Design review of the part built by this model. Coordinates are the model's own, in mm. Face numbers are marked on the shaded views. A direction names the side the tool comes from. Round coordinates to 2 decimals unless told otherwise and drop trailing zeros. Order: outer loops, then holes, each group sorted by start corner. A loop starts at its lowest first (then second) coordinate and runs counter-clockwise, first axis right, second up. Notation, with made-up numbers: (-29, 19.5) - (23, 19.5) arc R11 cw to (23, 35.5) - close; hole circle Ø8 at (49.5, 41). An arc over 180 degrees is marked (long way). Write item = value, one per line.
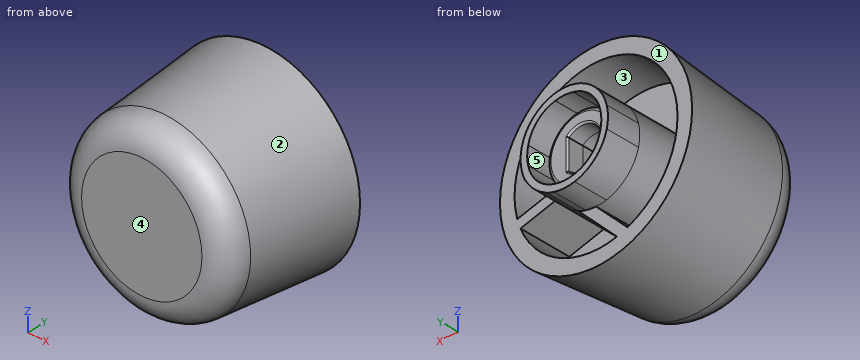
from build123d import *
from build123d.topology import SkipClean

# Parameters (mm, degrees)
SKETCH1_R             = 5
BOSS_EXTRUDE1_DEPTH   = 2.5
BOSS_EXTRUDE2_DEPTH   = 5.2
BOSS_EXTRUDE2_2_DEPTH = 5.2
BOSS_EXTRUDE2_3_DEPTH = 5.2
BOSS_EXTRUDE2_4_DEPTH = 5.2
FILLET1_R             = 0.5
FILLET2_R             = 0.5
FILLET3_R             = 0.5
FILLET4_R             = 0.5
SKETCH3_R             = 14.5
BOSS_EXTRUDE3_DEPTH   = 20
SKETCH4_OUTSIDE_W     = 44.126
SKETCH4_OUTSIDE_H     = 44.126
SKETCH4_OUTSIDE_R     = 14.5
CUT_EXTRUDE2_DEPTH    = 20
CUT_EXTRUDE2_DRAFT    = 5
FILLET5_R             = 4
CUT_EXTRUDE3_START    = -14
CUT_EXTRUDE3_DEPTH    = 14
FILLET6_R             = 0.25
FILLET7_R             = 0.5
CUT_EXTRUDE4_START    = -8
SKETCH6_R             = 12.3
SKETCH6_R_2           = 6.6
CUT_EXTRUDE4_DEPTH    = 8
BOSS_EXTRUDE4_DEPTH   = 8
BOSS_EXTRUDE5_DEPTH   = 5.2


# Read off the part's stored shape, not the designer's step: Boss-Extrude5
with BuildPart() as part:
    # Sketch1 → Boss-Extrude1 (new body)
    with BuildSketch(Plane(origin=(0, 0, 0), x_dir=(1, 0, 0), z_dir=(0, 1, 0))):
        with Locations(Location((0, 0, 0), (0, 0, 270))):
            Circle(SKETCH1_R)
        with BuildLine():
            Line((2, 2.236067977), (2, -2.236067977))
            ThreePointArc((2, -2.236067977), (-3, 0), (2, 2.236067977))
        make_face(mode=Mode.SUBTRACT)
    extrude(amount=BOSS_EXTRUDE1_DEPTH)



with BuildPart() as body_2:
    # Sketch2 → Boss-Extrude2 (new body)
    with BuildSketch(Plane.XZ):
        with BuildLine():
            Line((-6.305354867, 1.95), (-5.249523788, 1.95))
            ThreePointArc((-5.249523788, 1.95), (-5.6, 0), (-5.249523788, -1.95))
            Line((-5.249523788, -1.95), (-6.305354867, -1.95))
            ThreePointArc((-6.305354867, -1.95), (-6.6, 0), (-6.305354867, 1.95))
        make_face()
    extrude(amount=-BOSS_EXTRUDE2_DEPTH)

    # Fillet4
    fillet4_edges = [body_2.edges().sort_by_distance(p)[0] for p in [
        (-6.305354867, 2.6, 1.95),
        (-5.249523788, 2.6, -1.95),
        (-6.305354867, 2.6, -1.95),
        (-5.249523788, 2.6, 1.95),
    ]]
    fillet(fillet4_edges, radius=FILLET4_R - 0.0001)  # a hair under: the kernel refuses the full size


with BuildPart() as body_3:
    # Sketch2 → Boss-Extrude2 2 (new body)
    with BuildSketch(Plane.XZ):
        with BuildLine():
            Line((-1.95, 6.305354867), (-1.95, 5.249523788))
            ThreePointArc((-1.95, 5.249523788), (0, 5.6), (1.95, 5.249523788))
            Line((1.95, 5.249523788), (1.95, 6.305354867))
            ThreePointArc((1.95, 6.305354867), (0, 6.6), (-1.95, 6.305354867))
        make_face()
    extrude(amount=-BOSS_EXTRUDE2_2_DEPTH)

    # Fillet3
    fillet3_edges = [body_3.edges().sort_by_distance(p)[0] for p in [
        (-1.95, 2.6, 6.305354867),
        (-1.95, 2.6, 5.249523788),
        (1.95, 2.6, 6.305354867),
        (1.95, 2.6, 5.249523788),
    ]]
    fillet(fillet3_edges, radius=FILLET3_R - 0.0001)  # a hair under: the kernel refuses the full size


with BuildPart() as body_4:
    # Sketch2 → Boss-Extrude2 3 (new body)
    with BuildSketch(Plane.XZ):
        with BuildLine():
            Line((6.305354867, 1.95), (5.249523788, 1.95))
            ThreePointArc((5.249523788, 1.95), (5.6, 0), (5.249523788, -1.95))
            Line((5.249523788, -1.95), (6.305354867, -1.95))
            ThreePointArc((6.305354867, -1.95), (6.6, 0), (6.305354867, 1.95))
        make_face()
    extrude(amount=-BOSS_EXTRUDE2_3_DEPTH)

    # Fillet2
    fillet2_edges = [body_4.edges().sort_by_distance(p)[0] for p in [
        (6.305354867, 2.6, 1.95),
        (6.305354867, 2.6, -1.95),
        (5.249523788, 2.6, -1.95),
        (5.249523788, 2.6, 1.95),
    ]]
    fillet(fillet2_edges, radius=FILLET2_R - 0.0001)  # a hair under: the kernel refuses the full size


with BuildPart() as body_5:
    # Sketch2 → Boss-Extrude2 4 (new body)
    with BuildSketch(Plane.XZ):
        with BuildLine():
            Line((1.95, -6.305354867), (1.95, -5.249523788))
            ThreePointArc((1.95, -5.249523788), (0, -5.6), (-1.95, -5.249523788))
            Line((-1.95, -5.249523788), (-1.95, -6.305354867))
            ThreePointArc((-1.95, -6.305354867), (0, -6.6), (1.95, -6.305354867))
        make_face()
    extrude(amount=-BOSS_EXTRUDE2_4_DEPTH)

    # Fillet1
    fillet1_edges = [body_5.edges().sort_by_distance(p)[0] for p in [
        (1.95, 2.6, -6.305354867),
        (-1.95, 2.6, -6.305354867),
        (1.95, 2.6, -5.249523788),
        (-1.95, 2.6, -5.249523788),
    ]]
    fillet(fillet1_edges, radius=FILLET1_R - 0.0001)  # a hair under: the kernel refuses the full size


with BuildPart() as part_1:
    add(part.part)

    add(body_2.part)  # Boss-Extrude3 merges body 2

    add(body_3.part)  # Boss-Extrude3 merges body 3

    add(body_4.part)  # Boss-Extrude3 merges body 4

    add(body_5.part)  # Boss-Extrude3 merges body 5
    # Sketch3 → Boss-Extrude3 (add)
    with BuildSketch(Plane(origin=(0, 0, 0), x_dir=(1, 0, 0), z_dir=(0, 1, 0))):
        with Locations(Location((0, 0, 0), (0, 0, 270))):
            Circle(SKETCH3_R)
    extrude(amount=-BOSS_EXTRUDE3_DEPTH)


with BuildPart() as cut_extrude2_tool:
    # Sketch4 outside → Cut-Extrude2 (with draft: the straight prism first)
    with BuildSketch(Plane(origin=(0, 0, 0), x_dir=(1, 0, 0), z_dir=(0, 1, 0))):
        Rectangle(SKETCH4_OUTSIDE_W, SKETCH4_OUTSIDE_H)
        Circle(SKETCH4_OUTSIDE_R, mode=Mode.SUBTRACT)
    extrude(amount=-CUT_EXTRUDE2_DEPTH)
    # Cut-Extrude2: the draft: its side faces are tilted about the plane it starts from
    cut_extrude2_sides = [cut_extrude2_tool.faces().sort_by_distance(p)[0] for p in [
        (0, -10, 22.063),
        (22.063, -10, 0),
        (0, -10, -22.063),
        (-22.063, -10, 0),
        (-14.5, -10, 0),
    ]]
    draft(cut_extrude2_sides, Plane(origin=(0, 0, 0), x_dir=(1, 0, 0), z_dir=(0, 1, 0)), CUT_EXTRUDE2_DRAFT)


with BuildPart() as part_2:
    add(part_1.part)

    # Cut-Extrude2: cut by cut_extrude2_tool
    add(cut_extrude2_tool.part, mode=Mode.SUBTRACT)

    # Fillet5
    fillet5_edges = [part_2.edges().sort_by_distance(p)[0] for p in [
        (-12.750226729, -20, 0),
    ]]
    fillet(fillet5_edges, radius=FILLET5_R)

    # Sketch5 → Cut-Extrude3 (cut)
    with SkipClean():  # the faces are left unmerged after this step: merging them gives an invalid solid
        with BuildSketch(Plane(origin=(0, 0, 0), x_dir=(1, 0, 0), z_dir=(0, 1, 0)).offset(CUT_EXTRUDE3_START)):
            with BuildLine():
                Line((2, -2.236067977), (2, 2.236067977))
                ThreePointArc((2, 2.236067977), (-3, 0), (2, -2.236067977))
            make_face()
        extrude(amount=CUT_EXTRUDE3_DEPTH, mode=Mode.SUBTRACT)

    # Fillet6
    fillet6_edges = [part_2.edges().sort_by_distance(p)[0] for p in [
        (-3, 2.5, 0),
        (2, 2.5, 0),
    ]]
    fillet(fillet6_edges, radius=FILLET6_R)

    # Fillet7
    fillet7_edges = [part_2.edges().sort_by_distance(p)[0] for p in [
        (0, 2.5, -5),
    ]]
    fillet(fillet7_edges, radius=FILLET7_R)

    # Sketch6 → Cut-Extrude4 (cut)
    with SkipClean():  # the faces are left unmerged after this step: merging them gives an invalid solid
        with BuildSketch(Plane(origin=(0, 0, 0), x_dir=(1, 0, 0), z_dir=(0, 1, 0)).offset(CUT_EXTRUDE4_START)):
            with Locations(Location((0, 0, 0), (0, 0, 270))):
                Circle(SKETCH6_R)
            with Locations(Location((0, 0, 0), (0, 0, 76.248877743))):
                Circle(SKETCH6_R_2, mode=Mode.SUBTRACT)
        extrude(amount=CUT_EXTRUDE4_DEPTH, mode=Mode.SUBTRACT)

    # Sketch7 → Boss-Extrude4 (add)
    with SkipClean():  # the faces are left unmerged after this step: merging them gives an invalid solid
        with BuildSketch(Plane(origin=(0, -8, 0), x_dir=(1, 0, 0), z_dir=(0, 1, 0))):
            with BuildLine():
                Line((6.375110454, 1.708205698), (11.880887663, 3.183474255))
                ThreePointArc((11.880887663, 3.183474255), (11.664219973, 3.903328376), (11.40398128, 4.608601845))
                Line((11.40398128, 4.608601845), (5.820052572, 3.112392657))
                ThreePointArc((5.820052572, 3.112392657), (6.137868976, 2.426224317), (6.375110454, 1.708205698))
            make_face()
            with BuildLine():
                Line((2.697938648, 6.023381696), (-3.164606791, 11.885927135))
                ThreePointArc((-3.164606791, 11.885927135), (-3.964993354, 11.643402754), (-4.747049149, 11.347049149))
                Line((-4.747049149, 11.347049149), (0, 6.6))
                ThreePointArc((0, 6.6), (1.379434813, 6.454235787), (2.697938648, 6.023381696))
            make_face()
        extrude(amount=BOSS_EXTRUDE4_DEPTH)

    # Boss-Extrude5 outline → Boss-Extrude5 (add)
    with SkipClean():  # the faces are left unmerged after this step: merging them gives an invalid solid
        with BuildSketch(Plane(origin=(0, 0, 0), x_dir=(1, 0, 0), z_dir=(0, 1, 0))):
            with BuildLine():
                ThreePointArc((5.820052572, 3.112392657), (4.500834134, 4.827265489), (2.697938648, 6.023381696))
                Line((2.697938648, 6.023381696), (2.63830786, 6.083012483))
                ThreePointArc((2.63830786, 6.083012483), (2.110900212, 6.270800504), (1.568852459, 6.410826933))
                ThreePointArc((1.568852459, 6.410826933), (1.84333588, 6.233843964), (1.95, 5.925158226))
                ThreePointArc((1.95, 5.925158226), (1.772102461, 5.542731755), (1.36499998, 5.432436198))
                ThreePointArc((1.36499998, 5.432436198), (4.001957645, 4.001957645), (5.432436198, 1.36499998))
                ThreePointArc((5.432436198, 1.36499998), (5.542731755, 1.772102461), (5.925158226, 1.95))
                ThreePointArc((5.925158226, 1.95), (6.233843964, 1.84333588), (6.410826933, 1.568852459))
                ThreePointArc((6.410826933, 1.568852459), (6.393348383, 1.638626394), (6.375110454, 1.708205698))
                Line((6.375110454, 1.708205698), (6.379456664, 1.709370261))
                ThreePointArc((6.379456664, 1.709370261), (6.162816143, 2.431981568), (5.861013343, 3.123368063))
                Line((5.861013343, 3.123368063), (5.820052572, 3.112392657))
            make_face()
            with BuildLine():
                ThreePointArc((-1.95, 5.925158226), (-1.84333588, 6.233843964), (-1.568852459, 6.410826933))
                ThreePointArc((-1.568852459, 6.410826933), (-4.666904756, 4.666904756), (-6.410826932, 1.568852459))
                ThreePointArc((-6.410826932, 1.568852459), (-6.233843964, 1.84333588), (-5.925158226, 1.95))
                ThreePointArc((-5.925158226, 1.95), (-5.542731755, 1.772102461), (-5.432436198, 1.36499998))
                ThreePointArc((-5.432436198, 1.36499998), (-4.001957645, 4.001957645), (-1.36499998, 5.432436198))
                ThreePointArc((-1.36499998, 5.432436198), (-1.772102461, 5.542731755), (-1.95, 5.925158226))
            make_face()
            with BuildLine():
                ThreePointArc((-5.925158226, -1.95), (-6.233843964, -1.84333588), (-6.410826933, -1.568852459))
                ThreePointArc((-6.410826933, -1.568852459), (-4.666904756, -4.666904756), (-1.568852459, -6.410826933))
                ThreePointArc((-1.568852459, -6.410826933), (-1.84333588, -6.233843964), (-1.95, -5.925158226))
                ThreePointArc((-1.95, -5.925158226), (-1.772102461, -5.542731755), (-1.36499998, -5.432436198))
                ThreePointArc((-1.36499998, -5.432436198), (-4.001957645, -4.001957645), (-5.432436198, -1.36499998))
                ThreePointArc((-5.432436198, -1.36499998), (-5.542731755, -1.772102461), (-5.925158226, -1.95))
            make_face()
            with BuildLine():
                ThreePointArc((1.568852459, -6.410826933), (4.666904756, -4.666904756), (6.410826933, -1.568852459))
                ThreePointArc((6.410826933, -1.568852459), (6.233843964, -1.84333588), (5.925158226, -1.95))
                ThreePointArc((5.925158226, -1.95), (5.542731755, -1.772102461), (5.432436198, -1.36499998))
                ThreePointArc((5.432436198, -1.36499998), (4.001957645, -4.001957645), (1.36499998, -5.432436198))
                ThreePointArc((1.36499998, -5.432436198), (1.772102461, -5.542731755), (1.95, -5.925158226))
                ThreePointArc((1.95, -5.925158226), (1.84333588, -6.233843964), (1.568852459, -6.410826933))
            make_face()
        extrude(amount=BOSS_EXTRUDE5_DEPTH)


solid = part_2.part
1) For the marked faces 4 and 5, list the 3-axis set-ups (+Z, -Z, +X, -X, +Y, -Y) from which the entire face can be reached by the end or side of a thin tool; tool diameter is ignored.
Findings:
face_4 = +Z, -Z, +X, -X, -Y
face_5 = +Y
2) To check wall thickness, follow L1, parallel to X at y = 1.5, z = 0; L2, parallel to X at y = -0.25, z = -7.5; L3, parallel to Z at x = -1.5, y = -4. State the ranges of each line that lie inside material, in increasing order. Write a range as from..to.
Findings:
L1 = -6.6..-5.6, -5..-3, 2..5, 5.6..6.6
L2 = -12.38..-9.75, -0.9..1.22, 9.75..12.38
L3 = -14.07..-12.21, -10.22..-8.1, -6.43..-2.6, 2.6..6.43, 12.21..14.07
3) Clearance check with flat-ended pins moving along their axes: pin 1 Ø1.5 at (y, z) = (1.5, -6.5) entering from -X; pin 2 Ø4 at (x, y) = (-1, -10) entering from -Z; pin 3 Ø1.5 at (y, z) = (-4.5, -2) entering from -X. State where each tip first meets the part, or that it passes through.
Findings:
pin_1 = -3.24
pin_2 = -13.79
pin_3 = -14.08
4) We need section B-B on y = -18.25. Write out the cut boundary in (x, z), and give its area (3 significant figures).
Findings:
outline = circle Ø24.78 at (0, 0)
area = 482 mm^2
5) The part is to be moulded in two halves that separate along X. For the marked faces 1, 2 and 3, say which applies: released by +X, released by -X, zero draft, split by the parting line, or undercut.
Findings:
face_1 = zero draft
face_2 = split by the parting line
face_3 = undercut
